from build123d import *

# Parameters (mm, degrees)
ESQUISSE1_R                  = 1
BOSS_EXTRU_1_DEPTH           = 15
ENL_V_MAT_EXTRU_1_DEPTH      = 10
ENL_V_MAT_EXTRU_1_DEPTH_BACK = 10
ESQUISSE4_W                  = 0.167865562
ESQUISSE4_H                  = 1.310923544


with BuildPart() as part:
    # Esquisse1 → Boss.-Extru.1 (new body)
    with BuildSketch(Plane.XY):
        Circle(ESQUISSE1_R)
    extrude(amount=BOSS_EXTRU_1_DEPTH)

    # Esquisse2 → Révolution1 (revolve)
    with BuildSketch(Plane(origin=(0, 0, 0), x_dir=(1, 0, 0), z_dir=(0, 1, 0))):
        with BuildLine():
            Line((0, 0), (0, 1.5))
            ThreePointArc((0, 1.5), (1.060660172, 1.060660172), (1.5, 0))
            Line((1.5, 0), (0, 0))
        make_face()
    revolve(axis=Axis((0, 0, 0), (0, 0, -1)))

    # Esquisse4 → Enlèv. mat.-Extru.1 (cut, two sides: drawn at the far end of the back side and taken through both)
    with BuildSketch(Plane(origin=(0, 0, 0), x_dir=(1, 0, 0), z_dir=(0, 1, 0)).offset(-ENL_V_MAT_EXTRU_1_DEPTH_BACK)):
        with Locations((0, 1.5)):
            Rectangle(ESQUISSE4_W, ESQUISSE4_H)
    extrude(amount=ENL_V_MAT_EXTRU_1_DEPTH + ENL_V_MAT_EXTRU_1_DEPTH_BACK, mode=Mode.SUBTRACT)


solid = part.part
CAD build for the part. Positions are in the model's coordinates, mm. A direction names the side the tool comes from. Give positions to 0.01 mm unless a question says otherwise; leave off trailing zeros. Write each loop counter-clockwise with the first axis right and the second up, starting at its lowest first coordinate (ties: lowest second). Pieces come first, ordered by that corner, then holes. Notation, with made-up numbers: (21.5, 36.25) -> (46.5, 36.25) arc R12 ccw to (46.5, 47.25) -> close; hole circle Ø8 at (7.25, -17). An arc over 180 degrees is marked (long way). Return JSON: item names as keys, results as strings.
Item 1: Band-saw the part on D-D (x = -0.5). List the corners of the cut face in (y, z), then the cut area to 3 significant figures.
Answer below:
{"outline": "(-1.41, 0) arc R1.41 ccw to (1.41, 0) -> (0.87, 0) -> (0.87, 15) -> (-0.87, 15) -> (-0.87, 0) -> close", "area": "29.1 mm2"}
Item 2: Band-saw the part on C-C (x = 0.65). List the corners of the cut face in (y, z).
Answer below:
{"outline": "(-1.35, 0) arc R1.35 ccw to (1.35, 0) -> (0.76, 0) -> (0.76, 15) -> (-0.76, 15) -> (-0.76, 0) -> close"}
Item 3: Tool access for faces 1 (the flat face through (0, 0, 15)), 2 (the cylindrical face through (0, -1, 7)): list every direction of +Z, -Z, +X, -X, +Y, -Y with a clear straight run to the whole face (end or side of a thin tool).
Answer below:
{"face 1": "+Z, +X, -X, +Y, -Y", "face 2": "+Z"}
Item 4: Band-saw the part on A-A (y = 0). List the corners of the cut face in (x, z).
Answer below:
{"outline": "(-1.5, 0) arc R1.5 ccw to (-0.08, -1.5) -> (-0.08, -0.84) -> (0.08, -0.84) -> (0.08, -1.5) arc R1.5 ccw to (1.5, 0) -> (1, 0) -> (1, 15) -> (-1, 15) -> (-1, 0) -> close"}
Item 5: Drop flat-ended pins along their axis: pin 1 (1 mm diameter, centred on x = 0.5, y = 1, fed in from -Z); pin 2 (1.5 mm diameter, centred on x = -1, y = 0, fed in from -Z). Give the stop position or say it passes through.
Answer below:
{"pin 1": "stops at z = -1.37", "pin 2": "stops at z = -1.48"}
Item 6: Drill centre lines: probe 1 along X at (y, z) = (0.05, 8); probe 2 along Y at (x, z) = (-0.65, 9.5); probe 3 along Z at (x, y) = (-0.25, -0.2). Where is each one in solid material? Low to high.
Answer below:
{"probe 1": "x = -1 to 1", "probe 2": "y = -0.76 to 0.76", "probe 3": "z = -1.47 to 15"}
Item 7: Band-saw the part on B-B (z = 3). List the corners of the cut face in (x, y), then the cut area to 3 significant figures.
Answer below:
{"outline": "circle Ø2 at (0, 0)", "area": "3.14 mm2"}
